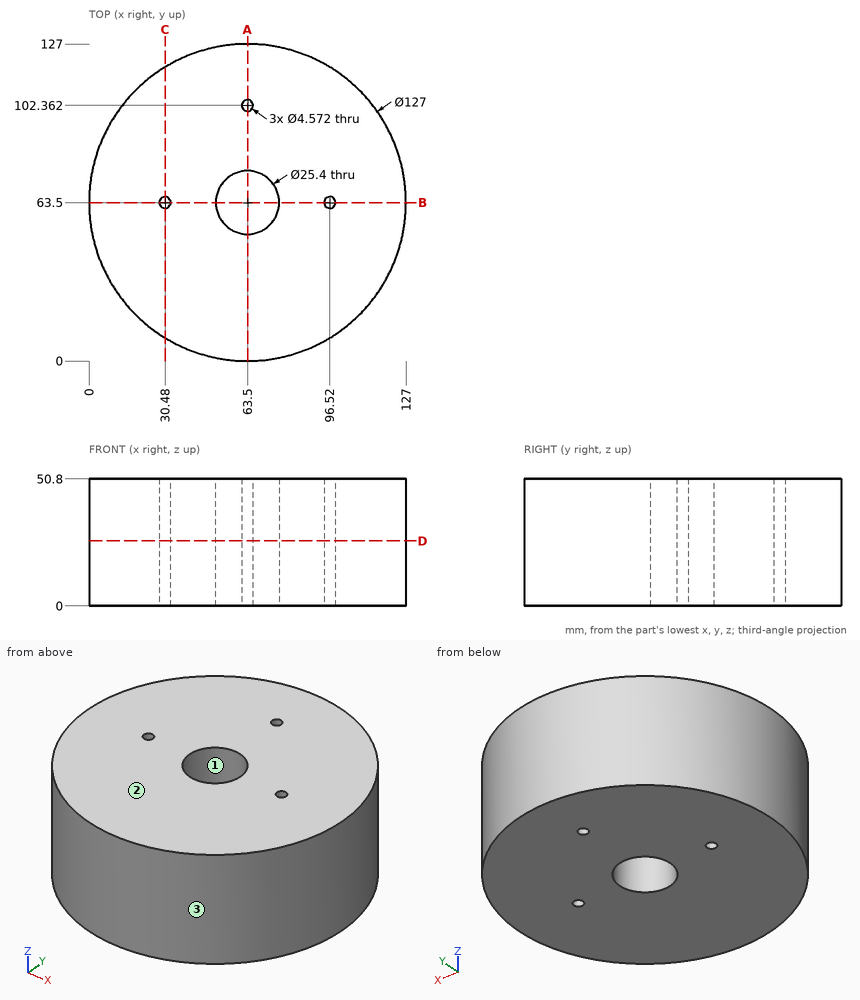
Here's the drawing with two shaded views (mm, measured from the low corner). I have some questions. Coordinates: 2 decimals unless noted, no trailing zeros. Write each loop counter-clockwise with the first axis right and the second up, starting at its lowest first coordinate (ties: lowest second). Pieces come first, ordered by that corner, then holes. Notation, with made-up numbers: M -15.75,34 L 14.25,34 A20 cw 14.25,72 Z; hole C 54,17 d8. An arc over 180 degrees is marked long. Use one line per item in the form item = value.
Q1. I need wall thicknesses on line 1 along Y through (x, z) = (63, 19); line 2 along Y through (x, z) = (30, 24); line 3 along Y through (x, z) = (30.48, 15.5). Which ranges of each line are inside material? Lowest first, please. Write a range as from..to.
Model answer:
line_1 = 0..50.81, 76.19..100.13, 104.59..127
line_2 = 9.56..61.26, 65.74..117.44
line_3 = 9.26..61.21, 65.79..117.74
Q2. If we section it at A-A (x = 63.5): Write out the boundary of the cut face in (y, z).
Model answer:
outline = M 0,0 L 50.8,0 L 50.8,50.8 L 0,50.8 Z; M 76.2,0 L 100.08,0 L 100.08,50.8 L 76.2,50.8 Z; M 104.65,0 L 127,0 L 127,50.8 L 104.65,50.8 Z
Q3. If we section it at C-C (x = 30.48): Write out the boundary of the cut face in (y, z).
Model answer:
outline = M 9.26,0 L 61.21,0 L 61.21,50.8 L 9.26,50.8 Z; M 65.79,0 L 117.74,0 L 117.74,50.8 L 65.79,50.8 Z
Q4. We'd pull the mould along Y, two halves only. Please class the marked faces 1, 2 and 3: +Y half, -Y half, draft (parallel to the pull), parting line (faces both ways), or undercut.
Model answer:
face_1 = undercut
face_2 = draft
face_3 = parting line
Q5. If we section it at B-B (y = 63.5): Write out the boundary of the cut face in (x, z), then the cut area to 3 significant figures.
Model answer:
outline = M 0,0 L 28.19,0 L 28.19,50.8 L 0,50.8 Z; M 32.77,0 L 50.8,0 L 50.8,50.8 L 32.77,50.8 Z; M 76.2,0 L 94.23,0 L 94.23,50.8 L 76.2,50.8 Z; M 98.81,0 L 127,0 L 127,50.8 L 98.81,50.8 Z
area = 4,700 mm^2
Q6. For P1, Ø12, axis at x = 72.5, z = 24.5, coming from the -Y side; P2, Ø8, axis at x = 87, z = 13.5, coming from the +Y side; P3, Ø6, axis at x = 37.5, y = 93, coming from the -Z side; P4, Ø4, axis at y = 45, z = 42, coming from the -X side, each with a flat end and sliding along its axis, tell me the tip position at first contact or that it passes through.
Model answer:
P1 = 0.07
P2 = 123.93
P3 = 0
P4 = 2.18
Q7. If we section it at D-D (z = 26): Write out the boundary of the cut face in (x, y), then the cut area to 3 significant figures.
Model answer:
outline = C 63.5,63.5 d127; hole C 30.48,63.5 d4.57; hole C 63.5,63.5 d25.4; hole C 63.5,102.36 d4.57; hole C 96.52,63.5 d4.57
area = 12,100 mm^2
